Part model, mm, in its own coordinate system. Give positions to 0.01 mm unless a question says otherwise; leave off trailing zeros. Loops run counter-clockwise (first coordinate to the right, second up) from the corner with the lowest first, then second, coordinate; pieces in that order, holes last. Notation, with made-up numbers: (-35.5, 83.25) -> (-18.5, 83.25) arc R10 ccw to (-18.5, 92.25) -> close; hole circle Ø11 at (-14, 35.25). An arc over 180 degrees is marked (long way). Write item = value, one per line.
Autodesk Inventor part; units mm, degrees
ref_plane "YZ Plane" through (0, 0, 0) normal (1, 0, 0) x (0, 1, 0)
ref_plane "XZ Plane" through (0, 0, 0) normal (0, 1, 0) x (-1, 0, 0)
ref_plane "XY Plane" through (0, 0, 0) normal (0, 0, 1) x (1, 0, 0)
sketch "Sketch1" plane through (0, 0, 0) normal (0, 0, 1) x (1, 0, 0)
  line L0 (0, 0) -> (0, 7.8365) construction
  line L1 (1.275, 0) -> (3.775, 0)
  line L2 (1.275, 0) -> (1.275, 8)
  line L3 (1.275, 8) -> (2.3, 8)
  line L4 (2.3, 8) -> (2.3, 15)
  line L5 (2.3, 15) -> (10, 15)
  arc A0 (10, 15) -> (3.775, 0) centre (24.9598, 0) ccw
  dimension "d0" = 1.275
  dimension "d1" = 15
  dimension "d2" = 8
  dimension "d3" = 2.3
  dimension "d4" = 10
  dimension "d5" = 2.5
revolve "Revolution1" add sketch "Sketch1" angle 360 about axis through (0, 0, 0) along (0, 1, 0)
fillet "Fillet1" radius 1 1 edges at (-3.775, 0, 0)
sketch "Sketch2" plane through (0, 15, 0) normal (0, 1, 0) x (1, 0, 0)
  circle A0 centre (0, 0) radius 2.3
  circle A1 centre (0, 0) radius 10
properties part number "knob_bottom"
1) Drill centre lines: line 1 along X through (y, z) = (1, 1); line 2 along Z through (x, y) = (0, 10.25); line 3 along Z through (x, y) = (0, 13). Where is each one in solid material? Low to high. Write a range as [from, to].
Resolved:
line_1 = [-3.66, -0.79], [0.79, 3.66]
line_2 = [-6.42, -2.3], [2.3, 6.42]
line_3 = [-8.23, -2.3], [2.3, 8.23]
2) Drop flat-ended pins along their axis: P1, Ø1.4, axis at x = -0.5, z = 0.5, coming from the +Y side; P2, Ø2, axis at x = 1.5, y = 10, coming from the +Z side; P3, Ø3, axis at y = 6.5, z = 0, coming from the +X side; P4, Ø7.5, axis at x = 0, z = 0, coming from the +Y side. Give the stop position or say it passes through.
Resolved:
P1 = 8
P2 = 6.72
P3 = 5.34
P4 = 15
3) Pull direction X, two halves, no side cores. Call faces 1 (the face through (2, 15, 2)), 2 (the face through (0.59, 4.06, 1.13)): pulls with the +X half, pulls with the -X half, needs draft (parallel to the pull), parting line crosses it, or undercut.
Resolved:
face_1 = needs draft
face_2 = undercut
4) Slice it at B-B, the plane y = 9.5. List the corners of the cut face in (x, z), and give its area (3 significant figures).
Resolved:
outline = circle Ø12.05 at (0, 0); hole circle Ø4.6 at (0, 0)
area = 97.4 mm²
